```python
from build123d import *


with BuildPart() as part:
    # Sketch1 → Revolve1 (revolve)
    with BuildSketch(Plane(origin=(0, 0, 0), x_dir=(0, 0, -1), z_dir=(1, 0, 0))):
        with BuildLine():
            Line((13.353, 4.905), (13.988, 4.905))
            ThreePointArc((13.988, 4.905), (14.526815367, 4.681815367), (14.75, 4.143))
            Line((14.75, 4.143), (14.75, 3.556))
            Line((14.75, 3.556), (14.369, 3.175))
            Line((14.369, 3.175), (0.25, 3.175))
            Line((0.25, 3.175), (0.25, 2.413))
            Line((0.25, 2.413), (0, 2.413))
            Line((0, 2.413), (0, 4.36))
            Line((0, 4.36), (1.638888889, 4.36))
            Line((1.638888889, 4.36), (3.526824269, 5.45))
            Line((3.526824269, 5.45), (12.337, 5.45))
            Line((12.337, 5.45), (12.337, 4.4145))
            Line((12.337, 4.4145), (13.353, 4.4145))
            Line((13.353, 4.4145), (13.353, 4.905))
        make_face()
    revolve1 = revolve(axis=Axis((0, 0, 0), (0, 0, -1)))

    # Mirror1: Revolve1 across plane
    add(revolve1.mirror(Plane.XY))


solid = part.part
```
Work out the finished part from the listing and answer in its coordinate system (mm). A direction names the side the tool comes from. Give positions to 0.01 mm unless a question says otherwise; leave off trailing zeros. Write each loop counter-clockwise with the first axis right and the second up, starting at its lowest first coordinate (ties: lowest second). Pieces come first, ordered by that corner, then holes.
(1) The mould has two halves that part along Z. Classify faces 4 (the cylindrical face through (0.2, -4.9, 13.7)), 5 (the cylindrical face through (4.377, -0.575, 12.852)): pulls with the +Z half, pulls with the -Z half, needs draft (parallel to the pull), parting line crosses it, or undercut.
Final values:
face 4: needs draft
face 5: undercut
(2) The part is cut by section A-A on z = 10. Write down the section's boundary in (x, y) (3 decimals).
Final values:
outline: circle Ø10.9 at (0, 0); hole circle Ø6.35 at (0, 0)
(3) Flat-ended cylindrical pins translate along their axes: pin 1 Ø5 at (x, y) = (-1.5, -0.5) entering from +Z; pin 2 Ø1.9 at (x, y) = (0.5, -1.5) entering from -Z; pin 3 Ø1.5 at (y, z) = (-2, -2.5) entering from +X; pin 4 Ø5 at (x, y) = (-1, 0) entering from -Z. Find the tip coordinate at first contact, or state that the pin passes through.
Final values:
pin 1: stops at z = 14.75
pin 2: stops at z = -0.25
pin 3: stops at x = 4.97
pin 4: stops at z = -14.69
(4) Which of the six approach directions +Z, -Z, +X, -X, +Y, -Y give full straight-line access (tool end or side, diameter ignored) to faces 1 (the cylindrical face through (-3.1, -0.69, -7.21)), 2 (the cylindrical face through (-3.1, -0.69, 7.21)), 3 (the cylindrical face through (4.377, -0.575, -12.852))?
Final values:
face 1: -Z
face 2: +Z
face 3: none
(5) Straight lines are drawn through the part: line 1 (X direction, y = 0, z = 0.1); line 2 (Z direction, x = 3.75, y = 2.75); line 3 (Z direction, x = 1, y = -2.25). For each, find the intervals that lie inside material, in ascending order.
Final values:
line 1: x = -4.36 to -2.41, 2.41 to 4.36
line 2: z = -14.56 to -13.35, -12.34 to -2.14, 2.14 to 12.34, 13.35 to 14.56
line 3: z = -0.25 to 0.25
(6) The part is cut by section B-B on z = -2.5. Write down the section's boundary in (x, y) (3 decimals), plus the area to 3 significant figures.
Final values:
outline: circle Ø9.714 at (0, 0); hole circle Ø6.35 at (0, 0)
area: 42.4 mm2
